```python
from build123d import *

# Parameters (mm, degrees)
CROQUIS1_R                 = 50
SALIENTE_EXTRUIR1_DEPTH    = 50
CROQUIS2_R                 = 25
SALIENTE_EXTRUIR2_DEPTH    = 800
CORTAR_EXTRUIR1_DEPTH      = 804.118920323
CORTAR_EXTRUIR1_DEPTH_BACK = 804.118920323
CROQUIS3_R                 = 50


with BuildPart() as part:
    # Croquis1 → Saliente-Extruir1 (new, symmetric)
    with BuildSketch(Plane(origin=(0, 0, 0), x_dir=(0, 0, -1), z_dir=(1, 0, 0))):
        Circle(CROQUIS1_R)
    extrude(amount=SALIENTE_EXTRUIR1_DEPTH, both=True)

    # Croquis2 → Saliente-Extruir2 (add)
    with BuildSketch(Plane(origin=(0, 0, 0), x_dir=(1, 0, 0), z_dir=(0, 1, 0))):
        with Locations(Location((0, 0, 0), (0, 0, 90))):
            Circle(CROQUIS2_R)
    extrude(amount=SALIENTE_EXTRUIR2_DEPTH)

    # Croquis3 → Cortar-Extruir1 (cut, two sides: drawn at the far end of the back side and taken through both)
    with BuildSketch(Plane(origin=(0, 0, 0), x_dir=(0, 0, -1), z_dir=(1, 0, 0)).offset(-CORTAR_EXTRUIR1_DEPTH_BACK)):
        with Locations((0, 830)):
            Circle(CROQUIS3_R)
    extrude(amount=CORTAR_EXTRUIR1_DEPTH + CORTAR_EXTRUIR1_DEPTH_BACK, mode=Mode.SUBTRACT)


solid = part.part
```
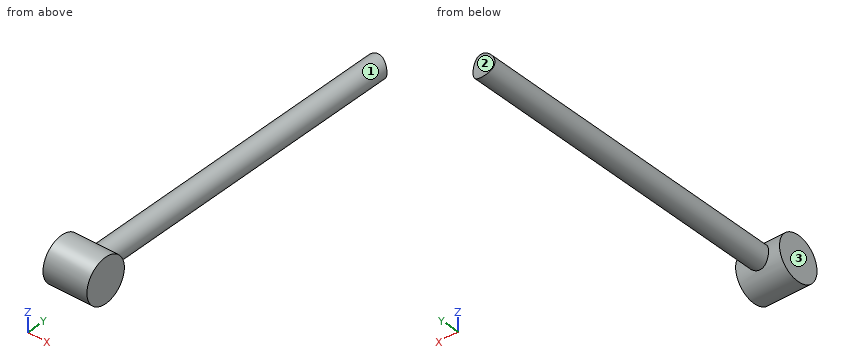
Work out the finished part from the listing and answer in its coordinate system (mm). Face numbers are marked on the shaded views. Round coordinates to 2 decimals unless told otherwise and drop trailing zeros. Write each loop counter-clockwise with the first axis right and the second up, starting at its lowest first coordinate (ties: lowest second). Pieces come first, ordered by that corner, then holes.
1) Flat-ended cylindrical pins translate along their axes: P1, Ø1, axis at x = 5, y = 520.5, coming from the +Z side; P2, Ø1, axis at y = 527.5, z = -18, coming from the +X side; P3, Ø5, axis at x = -11, z = -14.5, coming from the -Y side; P4, Ø12, axis at x = 33.5, y = 80.5, coming from the -Z side. Find the tip coordinate at first contact, or state that the pin passes through.
2) A cutting plane is placed at A-A on z = 0. Determine the outline of the cut face in (x, y).
3) A cutting plane is placed at D-D on x = -34. Determine the outline of the cut face in (y, z), and give its area (3 significant figures).
4) Consider probe 1 along Z at (x, y) = (-0.5, 476) (3 decimals); probe 2 along Z at (x, y) = (-2, 476). Determine where each line is inside the solid, lowest interval first.
5) A cutting plane is placed at C-C on y = 684. Determine the outline of the cut face in (x, z), and give its area (3 significant figures).
6) A cutting plane is placed at B-B on x = 0. Determine the outline of the cut face in (y, z).
7) Determine the mould class of the marked faces 1, 2 and 3 for opening direction Z: pulls with the +Z half, pulls with the -Z half, needs draft (parallel to the pull), parting line crosses it, or undercut.
Entries:
1. P1: stops at z = 24.59
1. P2: stops at x = 17.85
1. P3: stops at y = -48.54
1. P4: passes through
2. outline: (-50, -50) - (50, -50) - (50, 50) - (25, 50) - (25, 780) - (-25, 780) - (-25, 50) - (-50, 50) - close
3. outline: circle Ø100 at (0, 0)
3. area: 7,850 mm2
4. probe 1: z = -24.995 to 24.995
4. probe 2: z = -24.92 to 24.92
5. outline: circle Ø50 at (0, 0)
5. area: 1,960 mm2
6. outline: (43.3, -25) - (786.7, -25) arc R50 cw to (786.7, 25) - (43.3, 25) arc R50 ccw (long way) to start
7. face 1: parting line crosses it
7. face 2: undercut
7. face 3: needs draft
